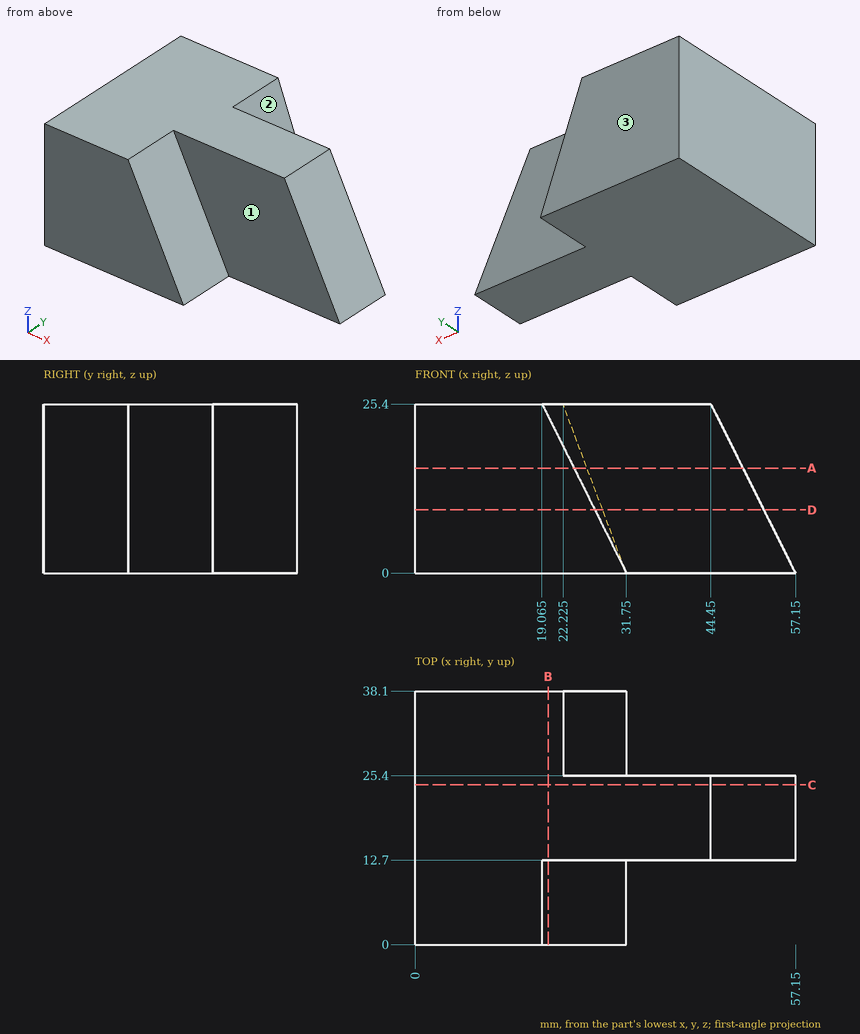
Study the drawing (mm; zero at the part's minimum x, y, z) and answer. A direction names the side the tool comes from. Coordinates: 2 decimals unless noted, no trailing zeros. Write each loop counter-clockwise with the first axis right and the second up, starting at its lowest first coordinate (ties: lowest second). Pieces come first, ordered by that corner, then holes. Notation, with made-up numbers: M -14.5,3.25 L -2.5,3.25 A17 cw -2.5,15.25 Z; hole C 8.5,31.25 d4. An arc over 180 degrees is marked long. Use a Markdown table: item, result. Add a question column.
1. Which of the six approach directions +Z, -Z, +X, -X, +Y, -Y give full straight-line access (tool end or side, diameter ignored) to the marked faces 1, 2 and 3?
2. Section D-D (z = 9.5) is taken. Give the vertices of the cut face in (x, y).
3. Straight lines are drawn through the part: line 1 along Y through (x, z) = (43, 21); line 2 along X through (y, z) = (36.5, 12); line 3 along X through (y, z) = (32, 4.75). For each, find the intervals that lie inside material, in ascending order. Write a range as [from, to].
4. Given P1, Ø12, axis at x = 44.5, z = 15.5, coming from the +Y side; P2, Ø6, axis at y = 19.5, z = 17.5, coming from the -X side; P3, Ø3, axis at y = 11, z = 15, coming from the +X side; P4, Ø12, axis at x = 44.5, z = 9, coming from the -Y side, each flat-ended and moving along its own axis, determine where each tip first touches the part or whether it passes through.
5. Section C-C (y = 24) is taken. Give the vertices of the cut face in (x, z), plus the area to 3 significant figures.
6. Section B-B (x = 20) is taken. Give the vertices of the cut face in (y, z), plus the area to 3 significant figures.
7. Section A-A (z = 15.75) is taken. Give the vertices of the cut face in (x, y) (1 decimal), plus the area to 3 significant figures.
Data:
| question | item | result |
|---|---|---|
| 1 | face 1 | +Z, +X, -Y |
| 1 | face 2 | +Z, +X, +Y |
| 1 | face 3 | +Z, -Z, +X, -X, +Y |
| 2 | outline | M 0,0 L 27.01,0 L 27.01,12.7 L 52.4,12.7 L 52.4,25.4 L 28.19,25.4 L 28.19,38.1 L 0,38.1 Z |
| 3 | line 1 | y = [12.7, 25.4] |
| 3 | line 2 | x = [0, 27.25] |
| 3 | line 3 | x = [0, 29.97] |
| 4 | P1 | stops at y = 25.4 |
| 4 | P2 | stops at x = 0 |
| 4 | P3 | stops at x = 25.01 |
| 4 | P4 | stops at y = 12.7 |
| 5 | outline | M 0,0 L 57.15,0 L 44.45,25.4 L 0,25.4 Z |
| 5 | area | 1,290 mm2 |
| 6 | outline | M 0,0 L 38.1,0 L 38.1,25.4 L 12.7,25.4 L 12.7,23.53 L 0,23.53 Z |
| 6 | area | 944 mm2 |
| 7 | outline | M 0,0 L 23.9,0 L 23.9,12.7 L 49.3,12.7 L 49.3,25.4 L 25.8,25.4 L 25.8,38.1 L 0,38.1 Z |
| 7 | area | 1,260 mm2 |
